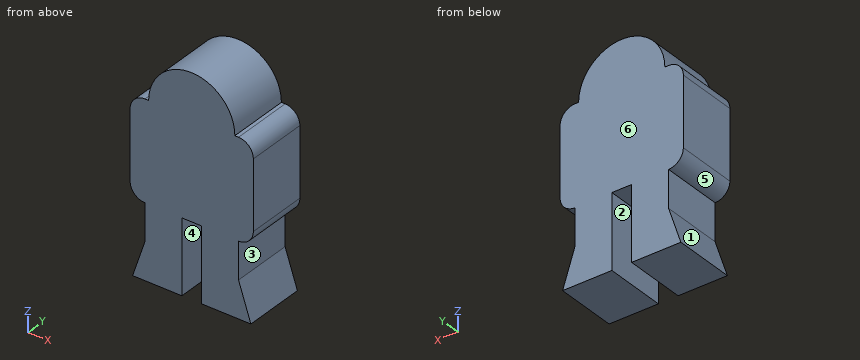
from build123d import *

# Parameters (mm, degrees)
F1_DEPTH = 25


with BuildPart() as f1:
    # F0 (on Front) → F1 (new body)
    with BuildSketch(Plane.XZ):
        with BuildLine():
            ThreePointArc((-25, -9), (-23.2426406871, -13.2426406871), (-19, -15))
            Line((-19, -15), (-4, -15))
            Line((-4, -15), (4, -15))
            Line((4, -15), (19, -15))
            ThreePointArc((19, -15), (23.2426406871, -13.2426406871), (25, -9))
            Line((25, -9), (25, 19))
            ThreePointArc((25, 19), (23.2426406871, 23.2426406871), (19, 25))
            Line((19, 25), (17.5, 25))
            ThreePointArc((17.5, 25), (0, 7.5), (-17.5, 25))
            Line((-17.5, 25), (-19, 25))
            ThreePointArc((-19, 25), (-23.2426406871, 23.2426406871), (-25, 19))
            Line((-25, 19), (-25, -9))
        make_face()
        Polygon((-4, -15), (-19, -15), (-19, -30), (-19, -45), (-4, -45), align=None)
        Polygon((-19, -45), (-19, -30), (-24, -45), align=None)
        Polygon((19, -15), (4, -15), (4, -45), (19, -45), (19, -30), align=None)
        Polygon((24, -45), (19, -30), (19, -45), align=None)
        with BuildLine():
            ThreePointArc((17.5, 25), (0, 42.5), (-17.5, 25))
            Line((-17.5, 25), (17.5, 25))
        make_face()
        with BuildLine():
            Line((17.5, 25), (-17.5, 25))
            ThreePointArc((-17.5, 25), (0, 7.5), (17.5, 25))
        make_face()
    extrude(amount=F1_DEPTH)


solid = f1.part
Source: CAD feature listing. Evaluate the final solid. Frame: model axes, mm. Face numbers are marked on the shaded views. A direction names the side the tool comes from. Coordinates: 2 decimals unless noted, no trailing zeros. Loops run counter-clockwise (first coordinate to the right, second up) from the corner with the lowest first, then second, coordinate; pieces in that order, holes last. Notation, with made-up numbers: M 5,39 L 9,39 A19 ccw 9,49 Z; hole C 76,-17 d11. An arc over 180 degrees is marked long. Answer in a Markdown table with one row per item.
Q1. Section B-B on y = -6. Return the cut outline in (x, z).
Answers below:
| item | result |
|---|---|
| outline | M -25,-9 A6 ccw -19,-15 L -19,-30 L -24,-45 L -4,-45 L -4,-15 L 4,-15 L 4,-45 L 24,-45 L 19,-30 L 19,-15 A6 ccw 25,-9 L 25,19 A6 ccw 19,25 L 17.5,25 A17.5 ccw -17.5,25 L -19,25 A6 ccw -25,19 Z |
Q2. Draft query along X for the marked faces 4, 5 and 6. Return one class per face: pulls with the +X half, pulls with the -X half, needs draft (parallel to the pull), parting line crosses it, or undercut.
Answers below:
| item | result |
|---|---|
| face 4 | undercut |
| face 5 | pulls with the -X half |
| face 6 | needs draft |
Q3. Ray query, probe 1 along X at (y, z) = (-3.75, -25.5); probe 2 along X at (y, z) = (-6.5, -31); probe 3 along Z at (x, y) = (3, -12.25). Return the intervals inside material, ascending. Write a range as from..to.
Answers below:
| item | result |
|---|---|
| probe 1 | x = -19..-4, 4..19 |
| probe 2 | x = -19.33..-4, 4..19.33 |
| probe 3 | z = -15..42.24 |
Q4. Section C-C on x = 0. Return the cut outline in (y, z), plus the area to 3 significant figures.
Answers below:
| item | result |
|---|---|
| outline | M -25,-15 L 0,-15 L 0,42.5 L -25,42.5 Z |
| area | 1,440 mm^2 |
Q5. Set-up query: the marked faces 1, 2 and 3. Return all of +Z, -Z, +X, -X, +Y, -Y with unobstructed straight access to the full face (end or side cutting, diameter ignored); none if empty.
Answers below:
| item | result |
|---|---|
| face 1 | -X, +Y, -Y |
| face 2 | -Z, +Y, -Y |
| face 3 | +X, +Y, -Y |
Q6. First-contact query: pin 1 (2 mm diameter, centred on x = 0, z = 32.5, fed in from +Y); pin 2 (4.5 mm diameter, centred on y = -18.5, z = -24, fed in from -X); pin 3 (2.5 mm diameter, centred on x = 2, y = -13.5, fed in from -Z); pin 4 (12.5 mm diameter, centred on y = -6.5, z = -27.5, fed in from +X). Flat tips, straight axial feed; report the tip coordinate or a pass-through.
Answers below:
| item | result |
|---|---|
| pin 1 | stops at y = 0 |
| pin 2 | stops at x = -19 |
| pin 3 | stops at z = -15 |
| pin 4 | stops at x = 20.25 |
Q7. Section D-D on z = 30. Return the cut outline in (x, y), plus the area to 3 significant figures.
Answers below:
| item | result |
|---|---|
| outline | M -16.77,-25 L 16.77,-25 L 16.77,0 L -16.77,0 Z |
| area | 839 mm^2 |
Q8. Section A-A on z = -24. Return the cut outline in (x, y).
Answers below:
| item | result |
|---|---|
| outline | M -19,-25 L -4,-25 L -4,0 L -19,0 Z; M 4,-25 L 19,-25 L 19,0 L 4,0 Z |
